For this review, use the dimensioned drawing (mm, ordinates from the lowest corner) and the shaded views. A direction names the side the tool comes from. Coordinates: 2 decimals unless noted, no trailing zeros. Order: outer loops, then holes, each group sorted by start corner. A loop starts at its lowest first (then second) coordinate and runs counter-clockwise, first axis right, second up. Notation, with made-up numbers: M 66,-4.5 L 90,-4.5 A11 ccw 90,11.5 Z; hole C 22,5.5 d3. An arc over 180 degrees is marked long. One line per item, written item: value.
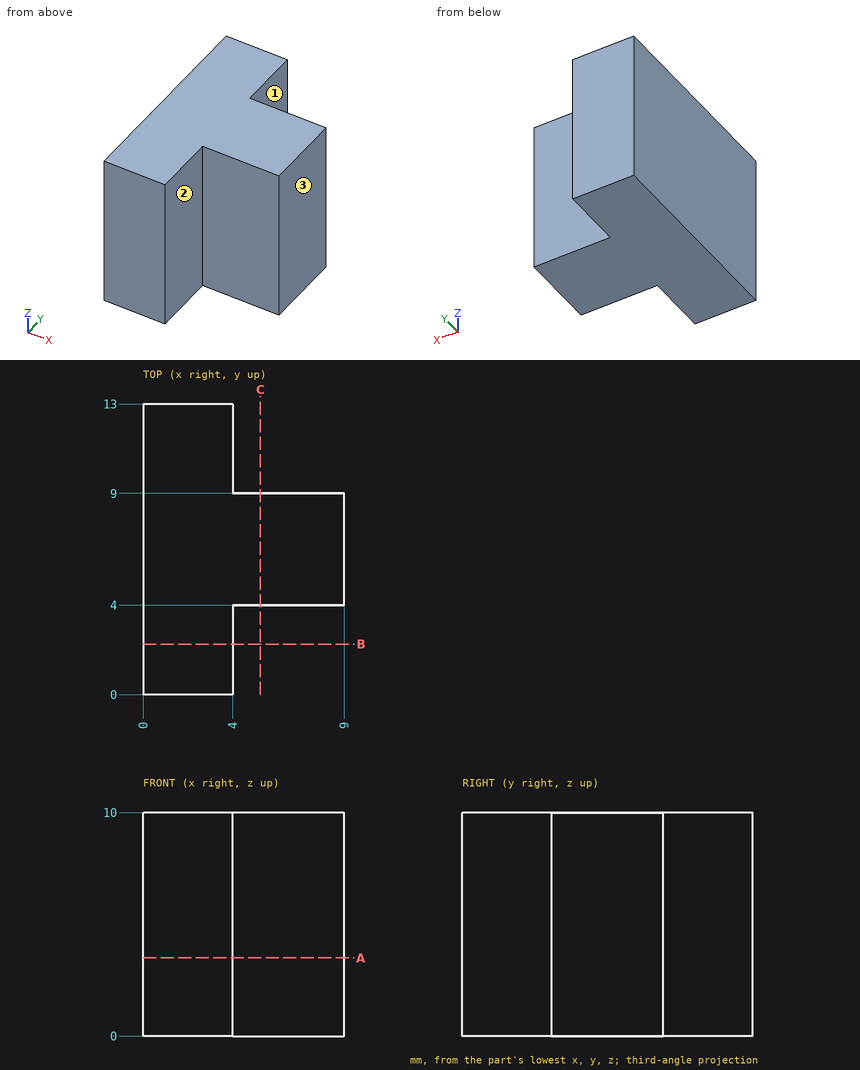
(1) For L1, parallel to X at y = 9.5, z = 5.25; L2, parallel to Y at x = 8, z = 1, list the stretches that pass through material, from the lowest coordinate up.
Geometry results:
L1: x = 0 to 4
L2: y = 4 to 9
(2) We need section B-B, the plane y = 2.25. State the section outline as (x, z) points.
Geometry results:
outline: M 0,0 L 4,0 L 4,10 L 0,10 Z
(3) We need section A-A, the plane z = 3.5. State the section outline as (x, y) points, plus the area to 3 significant figures.
Geometry results:
outline: M 0,0 L 4,0 L 4,4 L 9,4 L 9,9 L 4,9 L 4,13 L 0,13 Z
area: 77.0 mm2
(4) We need section C-C, the plane x = 5.25. State the section outline as (y, z) points, plus the area to 3 significant figures.
Geometry results:
outline: M 4,0 L 9,0 L 9,10 L 4,10 Z
area: 50.0 mm2
(5) Insertion check: pin 1 Ø4.5 at (y, z) = (2, 5) entering from +X; pin 2 Ø4 at (x, z) = (6.5, 5) entering from +Y; pin 3 Ø4.5 at (y, z) = (11.5, 4.5) entering from +X. Each pin has a flat end and moves straight along its axis. Give the tip position at first contact, or say it passes through.
Geometry results:
pin 1: stops at x = 9
pin 2: stops at y = 9
pin 3: stops at x = 4
(6) Tool access review of the marked faces 1, 2 and 3: name each direction out of +Z, -Z, +X, -X, +Y, -Y from which nothing blocks a thin tool from reaching the whole face with its end or side.
Geometry results:
face 1: +Z, -Z, +X, +Y
face 2: +Z, -Z, +X, -Y
face 3: +Z, -Z, +X, +Y, -Y
